Geometry check sheet. Reference: drawing and pictorial views, mm from the part's lowest x, y, z. Round coordinates to 2 decimals unless told otherwise and drop trailing zeros. Write each loop counter-clockwise with the first axis right and the second up, starting at its lowest first coordinate (ties: lowest second). Pieces come first, ordered by that corner, then holes. Notation, with made-up numbers: M 31.25,27 L 55.25,27 A18 ccw 55.25,32 Z; hole C -18,-21.5 d2. An arc over 180 degrees is marked long. Use a Markdown table: item, result. Add a question column.
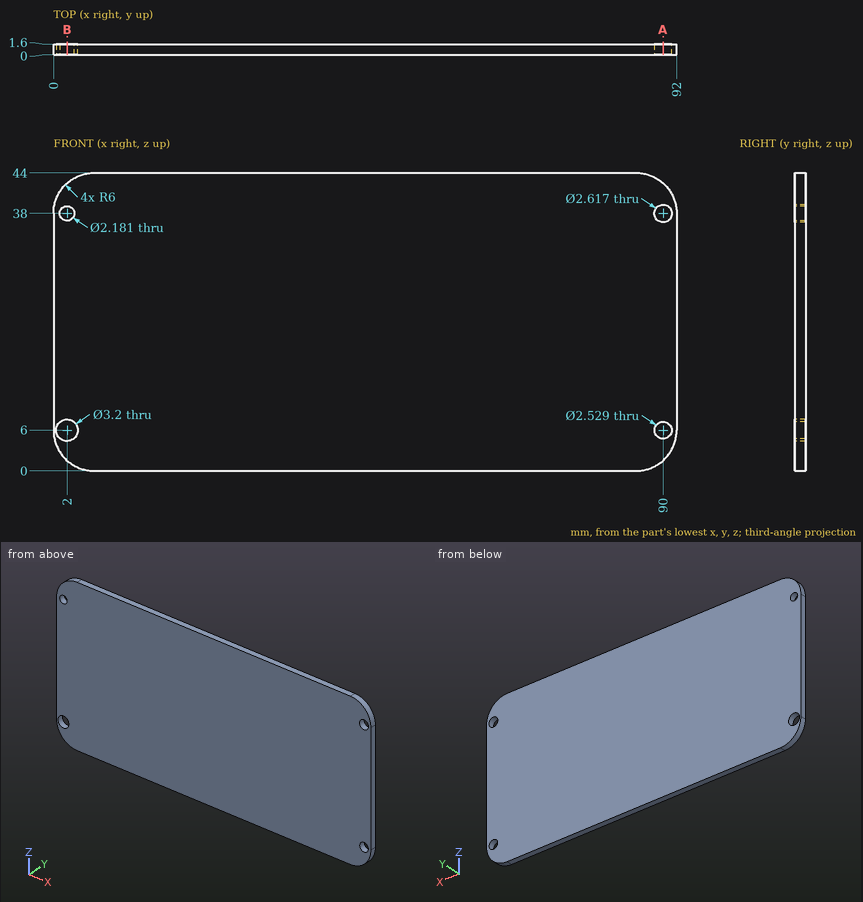
1. Cross-section at B-B on x = 2. Enter the section's corners in (y, z).
2. Scan lines: line 1 along X through (y, z) = (1.3, 6) (1 decimal); line 2 along X through (y, z) = (0.6, 38); line 3 along Z through (x, y) = (2, 0.6). Record each from-to range of solid material in increasing order. Write a range as from..to.
3. Cross-section at A-A on x = 90. Enter the section's corners in (y, z) (1 decimal).
4. Depth check by flat-ended pin: pin 1 Ø1.9 at (x, z) = (2, 6) entering from -Y. Enter the tip coordinate at first touch or a pass-through.
Answer:
| question | item | result |
|---|---|---|
| 1 | outline | M 0,1.53 L 1.6,1.53 L 1.6,4.4 L 0,4.4 Z; M 0,7.6 L 1.6,7.6 L 1.6,36.91 L 0,36.91 Z; M 0,39.09 L 1.6,39.09 L 1.6,42.47 L 0,42.47 Z |
| 2 | line 1 | x = 0..0.4, 3.6..88.7, 91.3..92 |
| 2 | line 2 | x = 0..0.91, 3.09..88.69, 91.31..92 |
| 2 | line 3 | z = 1.53..4.4, 7.6..36.91, 39.09..42.47 |
| 3 | outline | M 0,1.5 L 1.6,1.5 L 1.6,4.7 L 0,4.7 Z; M 0,7.3 L 1.6,7.3 L 1.6,36.7 L 0,36.7 Z; M 0,39.3 L 1.6,39.3 L 1.6,42.5 L 0,42.5 Z |
| 4 | pin 1 | passes through |
